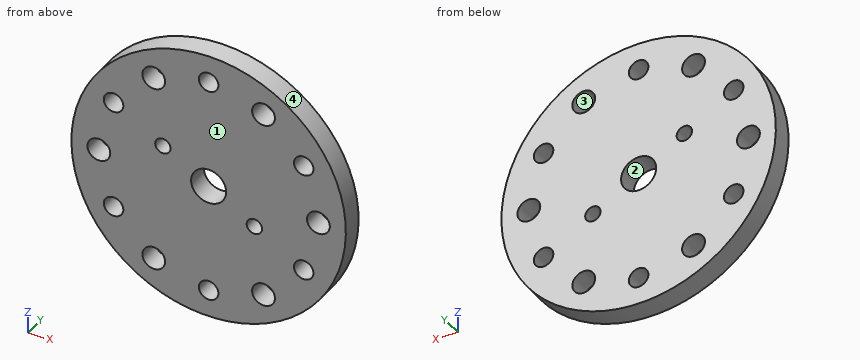
from build123d import *

# Parameters (mm, degrees)
SKETCH1_R                 = 15.875
BOSS_EXTRUDE1_DEPTH       = 2.54
TAP_DRILL_FOR_4_40_TAP1_D = 2.2606
CIRPATTERN1_COUNT         = 6
SKETCH8_R                 = 2.032
CUT_EXTRUDE1_DEPTH        = 2.54
SKETCH15_R                = 1.3208
CUT_EXTRUDE2_DEPTH        = 2.54
CIRPATTERN2_COUNT         = 6
F_2_56_TAPPED_HOLE1_D     = 1.778
F_2_56_TAPPED_HOLE2_D     = 1.778


with BuildPart() as part:
    # Sketch1 → Boss-Extrude1 (new body)
    with BuildSketch(Plane(origin=(0, 0, 0), x_dir=(1, 0, 0), z_dir=(0, 1, 0))):
        with Locations(Location((0, 0, 0), (0, 0, 270))):
            Circle(SKETCH1_R)
    extrude(amount=BOSS_EXTRUDE1_DEPTH)

    # Tap Drill for #4-40 Tap1 (through all)
    with Locations(Plane(origin=(0, 2.54, 0), x_dir=(1, 0, 0), z_dir=(0, 1, 0))):
        with Locations((0, 12.7)):
            tap_drill_for_4_40_tap1 = Hole(TAP_DRILL_FOR_4_40_TAP1_D / 2)

    # CirPattern1: Tap Drill for #4-40 Tap1 ×6 about axis
    cirpattern1_axis = Axis((0, 0, 0), (0, 1, 0))
    for i in range(1, CIRPATTERN1_COUNT):
        add(tap_drill_for_4_40_tap1.rotate(cirpattern1_axis, i * 360 / CIRPATTERN1_COUNT), mode=Mode.SUBTRACT)

    # Sketch8 → Cut-Extrude1 (cut)
    with BuildSketch(Plane(origin=(0, 2.54, 0), x_dir=(1, 0, 0), z_dir=(0, 1, 0))):
        with Locations(Location((0, 0, 0), (0, 0, 270))):
            Circle(SKETCH8_R)
    extrude(amount=-CUT_EXTRUDE1_DEPTH, mode=Mode.SUBTRACT)

    # Sketch15 → Cut-Extrude2 (cut)
    with BuildSketch(Plane(origin=(0, 2.54, 0), x_dir=(1, 0, 0), z_dir=(0, 1, 0))):
        with Locations(Location((12.7, 0, 0), (0, 0, 270))):
            Circle(SKETCH15_R)
    cut_extrude2 = extrude(amount=-CUT_EXTRUDE2_DEPTH, mode=Mode.SUBTRACT)

    # CirPattern2: Cut-Extrude2 ×6 about axis
    cirpattern2_axis = Axis((0, 0, 0), (0, 1, 0))
    for i in range(1, CIRPATTERN2_COUNT):
        add(cut_extrude2.rotate(cirpattern2_axis, i * 360 / CIRPATTERN2_COUNT), mode=Mode.SUBTRACT)

    # #2-56 Tapped Hole1 (through all)
    with Locations(Plane(origin=(0, 2.54, 0), x_dir=(1, 0, 0), z_dir=(0, 1, 0))):
        with Locations((-5.291415217, -3.055)):
            Hole(F_2_56_TAPPED_HOLE1_D / 2)

    # #2-56 Tapped Hole2 (through all)
    with Locations(Plane(origin=(0, 2.54, 0), x_dir=(1, 0, 0), z_dir=(0, 1, 0))):
        with Locations((5.291415217, 3.055)):
            Hole(F_2_56_TAPPED_HOLE2_D / 2)


solid = part.part
Build history of the part. All positions in model axes, mm. Face numbers are marked on the shaded views. Round coordinates to 2 decimals unless told otherwise and drop trailing zeros. Write each loop counter-clockwise with the first axis right and the second up, starting at its lowest first coordinate (ties: lowest second). Pieces come first, ordered by that corner, then holes. Notation, with made-up numbers: (-24, 17.5) - (4, 17.5) arc R5 ccw to (4, 23.5) - close; hole circle Ø3 at (5, 15.5). An arc over 180 degrees is marked (long way). One line per question, with ' | ' between items.
1. Mould opens along X. For the marked faces 1, 2, 3 and 4 say: released by +X, released by -X, zero draft, split by the parting line, or undercut.
Results are:
face 1: zero draft | face 2: undercut | face 3: undercut | face 4: split by the parting line
2. Drill centre lines: line 1 along X through (y, z) = (2.15, 0) (3 decimals); line 2 along Z through (x, y) = (12, 2.4); line 3 along X through (y, z) = (0.3, -12). Where is each one in solid material? Low to high. Write a range as from..to.
Results are:
line 1: -15.875..-14.021, -11.379..-2.032, 2.032..11.379, 14.021..15.875 | line 2: -10.39..-6.87, -5.83..-1.12, 1.12..5.83, 6.87..10.39 | line 3: -10.39..-7.21, -5.49..-0.89, 0.89..5.49, 7.21..10.39
3. Band-saw the part on B-B, the plane x = 1.5. Write the cut outline in (y, z).
Results are:
outline: (0, -15.8) - (2.54, -15.8) - (2.54, -1.37) - (0, -1.37) - close; (0, 1.37) - (2.54, 1.37) - (2.54, 15.8) - (0, 15.8) - close
4. Band-saw the part on C-C, the plane z = 6.35. Write the cut outline in (x, y).
Results are:
outline: (-14.55, 0) - (-12.13, 0) - (-12.13, 2.54) - (-14.55, 2.54) - close; (-9.87, 0) - (9.87, 0) - (9.87, 2.54) - (-9.87, 2.54) - close; (12.13, 0) - (14.55, 0) - (14.55, 2.54) - (12.13, 2.54) - close
5. Band-saw the part on A-A, the plane z = 0. Write the cut outline in (x, y) (3 decimals).
Results are:
outline: (-15.875, 0) - (-14.021, 0) - (-14.021, 2.54) - (-15.875, 2.54) - close; (-11.379, 0) - (-2.032, 0) - (-2.032, 2.54) - (-11.379, 2.54) - close; (2.032, 0) - (11.379, 0) - (11.379, 2.54) - (2.032, 2.54) - close; (14.021, 0) - (15.875, 0) - (15.875, 2.54) - (14.021, 2.54) - close
6. Drop flat-ended pins along their axis: pin 1 Ø1 at (x, y) = (-11, 0.5) entering from +Z; pin 2 Ø1.5 at (y, z) = (1, -8.5) entering from +X. Give the stop position or say it passes through.
Results are:
pin 1: z = 11.91 | pin 2: x = 13.85
7. Band-saw the part on D-D, the plane z = 12.7. Write the cut outline in (x, y) (3 decimals).
Results are:
outline: (-9.525, 0) - (-1.13, 0) - (-1.13, 2.54) - (-9.525, 2.54) - close; (1.13, 0) - (9.525, 0) - (9.525, 2.54) - (1.13, 2.54) - close
